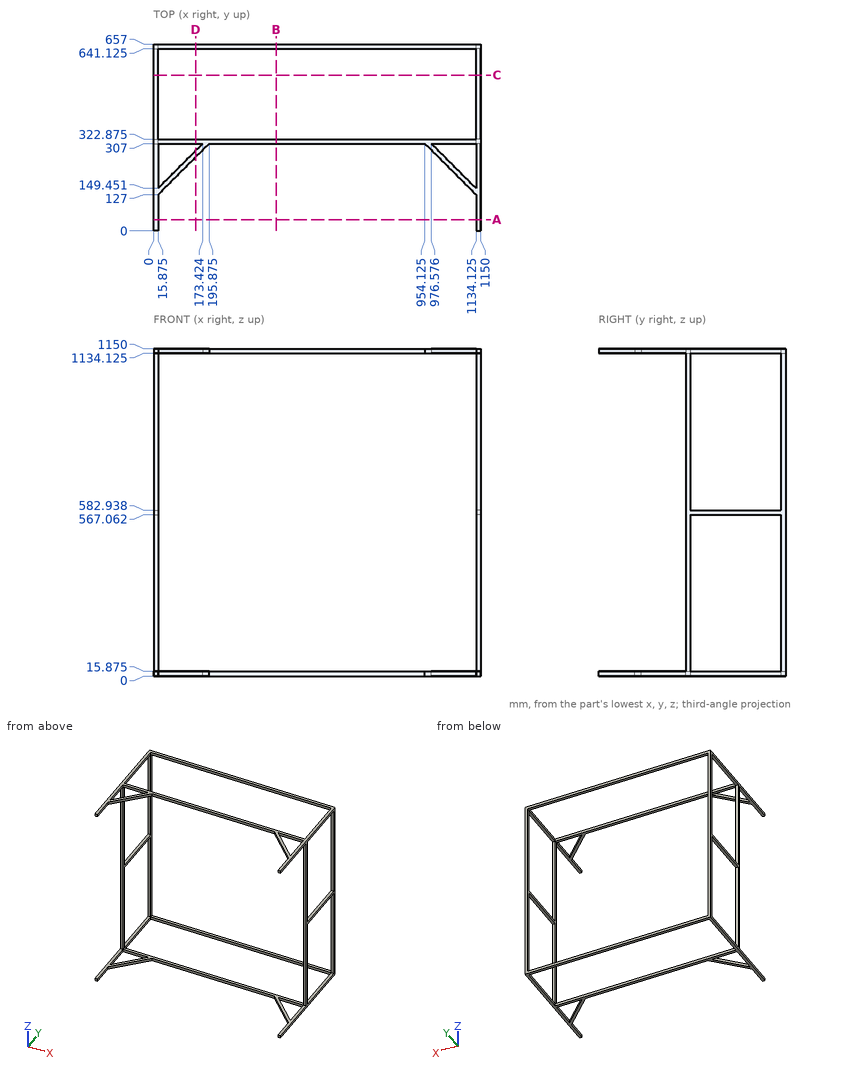
Answer from the drawing. Dimensions are ordinates in mm from the lowest x, y and z of the part. Give positions to 0.01 mm unless a question says otherwise; leave off trailing zeros. Loops run counter-clockwise (first coordinate to the right, second up) from the corner with the lowest first, then second, coordinate; pieces in that order, holes last.
Item 1: The part is cut by section C-C (y = 548). Write down the section's boundary in (x, z) (1 decimal), and give its area (3 significant figures).
Item 2: Find the intervals of material crossed by line 1 along X through (y, z) = (490, 570) (1 decimal), in increasing order.
Item 3: Each of these flat-tipped pins is pushed along its axis until it touches: pin 1 Ø17.5 at (x, z) = (513.5, 7) entering from -Y; pin 2 Ø8 at (x, z) = (1086.5, 1142.5) entering from -Y (1 decimal); pin 3 Ø8 at (x, z) = (92.5, 1144.5) entering from -Y (1 decimal). Where does it stop, or does it pass through?
Item 4: The part is cut by section B-B (x = 431.5). Write down the section's boundary in (y, z) (1 decimal).
Item 5: The part is cut by section A-A (y = 39.5). Write down the section's boundary in (x, z) (1 decimal).
Item 6: The part is cut by section D-D (x = 148.5). Write down the section's boundary in (y, z) (1 decimal).
Taken from the geometry:
1. outline: (0, 0) - (15.9, 0) - (15.9, 15.9) - (0, 15.9) - close; (0, 567.1) - (15.9, 567.1) - (15.9, 582.9) - (0, 582.9) - close; (0, 1134.1) - (15.9, 1134.1) - (15.9, 1150) - (0, 1150) - close; (1134.1, 0) - (1150, 0) - (1150, 15.9) - (1134.1, 15.9) - close; (1134.1, 567.1) - (1150, 567.1) - (1150, 582.9) - (1134.1, 582.9) - close; (1134.1, 1134.1) - (1150, 1134.1) - (1150, 1150) - (1134.1, 1150) - close
1. area: 1,510 mm2
2. line 1: x = 0 to 15.9, 1134.1 to 1150
3. pin 1: stops at y = 307
3. pin 2: stops at y = 170.6
3. pin 3: stops at y = 199.6
4. outline: (307, 0) - (322.9, 0) - (322.9, 15.9) - (307, 15.9) - close; (307, 1134.1) - (322.9, 1134.1) - (322.9, 1150) - (307, 1150) - close; (641.1, 0) - (657, 0) - (657, 15.9) - (641.1, 15.9) - close; (641.1, 1134.1) - (657, 1134.1) - (657, 1150) - (641.1, 1150) - close
5. outline: (0, 0) - (15.9, 0) - (15.9, 15.9) - (0, 15.9) - close; (0, 1134.1) - (15.9, 1134.1) - (15.9, 1150) - (0, 1150) - close; (1134.1, 0) - (1150, 0) - (1150, 15.9) - (1134.1, 15.9) - close; (1134.1, 1134.1) - (1150, 1134.1) - (1150, 1150) - (1134.1, 1150) - close
6. outline: (259.6, 0) - (282.1, 0) - (282.1, 15.9) - (259.6, 15.9) - close; (259.6, 1134.1) - (282.1, 1134.1) - (282.1, 1150) - (259.6, 1150) - close; (307, 0) - (322.9, 0) - (322.9, 15.9) - (307, 15.9) - close; (307, 1134.1) - (322.9, 1134.1) - (322.9, 1150) - (307, 1150) - close; (641.1, 0) - (657, 0) - (657, 15.9) - (641.1, 15.9) - close; (641.1, 1134.1) - (657, 1134.1) - (657, 1150) - (641.1, 1150) - close
